```python
from build123d import *

# Parameters (mm, degrees)
FILLET1_R          = 1
SKETCH2_R          = 8
CUT_EXTRUDE1_DEPTH = 4
SKETCH3_W          = 3
SKETCH3_H          = 2
CUT_REVOLVE1_ANGLE = 30
CIRPATTERN1_COUNT  = 6


with BuildPart() as part:
    # Sketch1 → Revolve1 (revolve)
    with BuildSketch(Plane.XY, mode=Mode.PRIVATE) as revolve1_sk:
        with BuildLine():
            Line((0, 0), (14, 0))
            Line((14, 0), (14, 1.5))
            Line((14, 1.5), (11.449688693, 1.949688693))
            Line((11.449688693, 1.949688693), (14.5, 5))
            add(Edge.make_bspline(
                [(11, 14), (11.868897118, 9.149631339), (14.5, 5)],
                knots=[0, 0, 0, 1, 1, 1], degree=2))
            Line((11, 14), (11, 16))
            add(Edge.make_bspline(
                [(9, 44), (6.119153374, 30.160071278), (11, 16)],
                knots=[0, 0, 0, 1, 1, 1], degree=2))
            Line((9, 44), (11, 45))
            Line((11, 45), (11, 55))
            Line((11, 55), (0, 55))
            Line((0, 55), (0, 0))
        make_face()
    revolve(revolve1_sk.sketch.rotate(Axis((0, 55, 0), (0, -1, 0)), 180), axis=Axis((0, 55, 0), (0, -1, 0)))

    # Fillet1
    fillet1_edges = [part.edges().sort_by_distance(p)[0] for p in [
        (14.5, 5, 0),
    ]]
    fillet(fillet1_edges, radius=FILLET1_R)

    # Sketch2 → Cut-Extrude1 (cut)
    with BuildSketch(Plane(origin=(0, 55, 0), x_dir=(1, 0, 0), z_dir=(0, 1, 0))):
        with Locations(Location((0, 0, 0), (0, 0, 180))):
            Circle(SKETCH2_R)
    extrude(amount=-CUT_EXTRUDE1_DEPTH, mode=Mode.SUBTRACT)

    # Sketch3 → Cut-Revolve1 (revolve, symmetric, cut)
    with BuildSketch(Plane.XY) as cut_revolve1_sk:
        with Locations((9.5, 54)):
            Rectangle(SKETCH3_W, SKETCH3_H)
    cut_revolve1 = revolve(axis=Axis((0, 0, 0), (0, 1, 0)), revolution_arc=CUT_REVOLVE1_ANGLE / 2, mode=Mode.SUBTRACT)
    cut_revolve1 = cut_revolve1 + revolve(cut_revolve1_sk.sketch, axis=Axis((0, 0, 0), (0, -1, 0)), revolution_arc=CUT_REVOLVE1_ANGLE / 2, mode=Mode.SUBTRACT)

    # CirPattern1: Cut-Revolve1 ×6 about axis
    cirpattern1_axis = Axis((0, 0, 0), (0, 1, 0))
    for i in range(1, CIRPATTERN1_COUNT):
        add(cut_revolve1.rotate(cirpattern1_axis, i * 360 / CIRPATTERN1_COUNT), mode=Mode.SUBTRACT)


solid = part.part
```
Read the model definition and answer for the solid it produces. Units are mm, in the model's axes. A direction names the side the tool comes from. Give positions to 0.01 mm unless a question says otherwise; leave off trailing zeros. Order: outer loops, then holes, each group sorted by start corner. A loop starts at its lowest first (then second) coordinate and runs counter-clockwise, first axis right, second up.
(1) For a pull along X with two mould halves and no side action, classify faces 4 (the cylindrical face through (-7.63, 53.03, 2.4)), 5 (the flat face through (-9.156, 54.014, -2.453)), 6 (the flat face through (8, 55, -5)) as released by +X, released by -X, zero draft, split by the parting line, or undercut.
(2) For faces 1 (the conical face through (-10.721, 2.106, 4.445)), 2 (the flat face through (7, 54, 7)), 3 (the flat face through (7, 54, -7)), determine the directions among +Z, -Z, +X, -X, +Y, -Y from which every point of the face is accessible in a straight line to the end or side of a thin tool.
(3) Find section A-A (y = 47). Give the vertices of the cut face in (x, z), plus the area to 3 significant figures.
(4) Given pin 1 (4 mm diameter, centred on x = 11, y = 5.5, fed in from +Z); pin 2 (2.5 mm diameter, centred on x = 6.5, z = -8.5, fed in from +Y); pin 3 (8 mm diameter, centred on y = 7.5, z = 8.5, fed in from -X), each flat-ended and moving along its own axis, determine where each tip first touches the part or whether it passes through.
(5) Straight lines are drawn through the part: L1, parallel to Z at x = 0, y = 54; L2, parallel to Y at x = -4.25, z = 5. For each, find the intervals that lie inside material, in ascending order.
Result sheet:
1. face 4: undercut
1. face 5: released by -X
1. face 6: zero draft
2. face 1: none
2. face 2: +Z, +Y
2. face 3: -Z, +Y
3. outline: circle Ø22 at (0, 0)
3. area: 380 mm2
4. pin 1: stops at z = 11.01
4. pin 2: stops at y = 53
4. pin 3: stops at x = -13.26
5. L1: z = -11 to -8, 8 to 11
5. L2: y = 0 to 51
